```python
from build123d import *

# Parameters (mm, degrees)
F1_DEPTH = 8


with BuildPart() as f1:
    # F0 (on Top) → F1 (new body)
    with BuildSketch(Plane.XY):
        with BuildLine():
            ThreePointArc((0, 14), (-9.899495, -9.899495), (14, 0))
            ThreePointArc((14, 0), (9.899495, 9.899495), (0, 14))
        make_face()
        with BuildLine():
            ThreePointArc((6.347522, 59.107844), (4.032635, 62.692937), (0, 64.089164))
            ThreePointArc((0, 64.089164), (-4.032635, 62.692937), (-6.347522, 59.107844))
            ThreePointArc((-6.347522, 59.107844), (-9.178693, 55.402974), (-13.333366, 53.286307))
            ThreePointArc((-13.333366, 53.286307), (-20.442135, 50.558658), (-24.717154, 44.257954))
            ThreePointArc((-24.717154, 44.257954), (-23.940515, 36.01526), (-18.369188, 29.891087))
            ThreePointArc((-18.369188, 29.891087), (-18.073469, 24.875996), (-22.751722, 26.70699))
            ThreePointArc((-22.751722, 26.70699), (-26.854522, 33.89811), (-34.453795, 37.18387))
            ThreePointArc((-34.453795, 37.18387), (-41.767174, 35.06511), (-46.558052, 29.147159))
            ThreePointArc((-46.558052, 29.147159), (-49.854987, 25.849917), (-54.253408, 24.302181))
            ThreePointArc((-54.253408, 24.302181), (-58.378374, 23.208447), (-60.952417, 19.804641))
            ThreePointArc((-60.952417, 19.804641), (-60.870679, 15.537919), (-58.176392, 12.228476))
            ThreePointArc((-58.176392, 12.228476), (-55.527732, 8.391005), (-54.798526, 3.785589))
            ThreePointArc((-54.798526, 3.785589), (-54.401108, -3.818141), (-49.729836, -9.830951))
            ThreePointArc((-49.729836, -9.830951), (-41.650573, -11.639455), (-34.104504, -8.233282))
            ThreePointArc((-34.104504, -8.233282), (-29.243487, -9.501785), (-32.430525, -13.38526))
            ThreePointArc((-32.430525, -13.38526), (-40.537522, -15.065076), (-46.01077, -21.277058))
            ThreePointArc((-46.01077, -21.277058), (-46.255668, -28.887228), (-42.107825, -35.272372))
            ThreePointArc((-42.107825, -35.272372), (-39.99077, -39.426847), (-39.877972, -44.08827))
            ThreePointArc((-39.877972, -44.08827), (-40.112455, -48.349328), (-37.670666, -51.849223))
            ThreePointArc((-37.670666, -51.849223), (-33.587513, -53.089975), (-29.607466, -51.55023))
            ThreePointArc((-29.607466, -51.55023), (-25.139332, -50.217048), (-20.533985, -50.946684))
            ThreePointArc((-20.533985, -50.946684), (-13.179599, -52.918399), (-6.017575, -50.333815))
            ThreePointArc((-6.017575, -50.333815), (-1.800955, -43.208839), (-2.708555, -34.979535))
            ThreePointArc((-2.708555, -34.979535), (0, -30.748422), (2.708555, -34.979535))
            ThreePointArc((2.708555, -34.979535), (1.800955, -43.208839), (6.017575, -50.333815))
            ThreePointArc((6.017575, -50.333815), (13.179599, -52.918399), (20.533985, -50.946684))
            ThreePointArc((20.533985, -50.946684), (25.139332, -50.217048), (29.607466, -51.55023))
            ThreePointArc((29.607466, -51.55023), (33.587513, -53.089975), (37.670666, -51.849223))
            ThreePointArc((37.670666, -51.849223), (40.112455, -48.349328), (39.877972, -44.08827))
            ThreePointArc((39.877972, -44.08827), (39.99077, -39.426847), (42.107825, -35.272372))
            ThreePointArc((42.107825, -35.272372), (46.255668, -28.887228), (46.01077, -21.277058))
            ThreePointArc((46.01077, -21.277058), (40.537522, -15.065076), (32.430525, -13.38526))
            ThreePointArc((32.430525, -13.38526), (29.243487, -9.501785), (34.104504, -8.233282))
            ThreePointArc((34.104504, -8.233282), (41.650573, -11.639455), (49.729836, -9.830951))
            ThreePointArc((49.729836, -9.830951), (54.401108, -3.818141), (54.798526, 3.785589))
            ThreePointArc((54.798526, 3.785589), (55.527732, 8.391005), (58.176392, 12.228476))
            ThreePointArc((58.176392, 12.228476), (60.870679, 15.537919), (60.952417, 19.804641))
            ThreePointArc((60.952417, 19.804641), (58.378374, 23.208447), (54.253408, 24.302181))
            ThreePointArc((54.253408, 24.302181), (49.854987, 25.849917), (46.558052, 29.147159))
            ThreePointArc((46.558052, 29.147159), (41.767174, 35.06511), (34.453795, 37.18387))
            ThreePointArc((34.453795, 37.18387), (26.854522, 33.89811), (22.751722, 26.70699))
            ThreePointArc((22.751722, 26.70699), (18.073469, 24.875996), (18.369188, 29.891087))
            ThreePointArc((18.369188, 29.891087), (23.940515, 36.01526), (24.717154, 44.257954))
            ThreePointArc((24.717154, 44.257954), (20.442135, 50.558658), (13.333366, 53.286307))
            ThreePointArc((13.333366, 53.286307), (9.178693, 55.402974), (6.347522, 59.107844))
        make_face()
        Polygon((-11.907824, -27.194431), (-13.235514, -39.826555), (-24.8391, -44.992804), (-35.114996, -37.526929), (-33.787306, -24.894804), (-22.18372, -19.728555), align=None, mode=Mode.SUBTRACT)
        with BuildLine():
            ThreePointArc((0, 14), (9.899495, 9.899495), (14, 0))
            ThreePointArc((14, 0), (-9.899495, -9.899495), (0, 14))
        make_face(mode=Mode.SUBTRACT)
        Polygon((22.18372, -19.728555), (33.787306, -24.894804), (35.114996, -37.526929), (24.8391, -44.992804), (13.235514, -39.826555), (11.907824, -27.194431), align=None, mode=Mode.SUBTRACT)
        Polygon((-29.54316, 2.921473), (-41.967304, 0.28064), (-50.466404, 9.719847), (-46.541361, 21.799887), (-34.117218, 24.44072), (-25.618117, 15.001513), align=None, mode=Mode.SUBTRACT)
        Polygon((6.350853, 29), (0, 29), (-6.350853, 29), (-12.701706, 40), (-6.350853, 51), (0, 51), (6.350853, 51), (12.701706, 40), align=None, mode=Mode.SUBTRACT)
        Polygon((25.618117, 15.001513), (34.117218, 24.44072), (46.541361, 21.799887), (50.466404, 9.719847), (41.967304, 0.28064), (29.54316, 2.921473), align=None, mode=Mode.SUBTRACT)
    extrude(amount=F1_DEPTH)


solid = f1.part
```
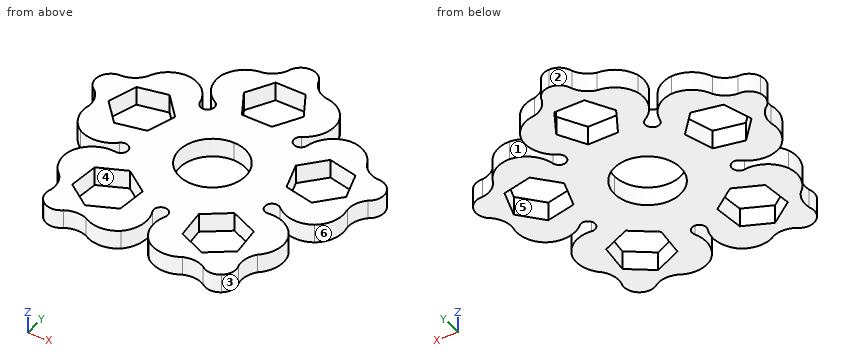
The listing builds one solid part. Answer for the finished solid, in the listing's coordinates (mm). Face numbers are marked on the shaded views. A direction names the side the tool comes from. Round coordinates to 2 decimals unless told otherwise and drop trailing zeros. Write each loop counter-clockwise with the first axis right and the second up, starting at its lowest first coordinate (ties: lowest second). Pieces come first, ordered by that corner, then holes. Notation, with made-up numbers: (64, 66.25) -> (123, 66.25) arc R7 cw to (123, 73.25) -> close; hole circle Ø2 at (85.5, 65). An arc over 180 degrees is marked (long way). Use CSV: the item, a comma, the result in double quotes. Start each with the question number.
(1) Each of these flat-tipped pins is pushed along its axis until it touches: pin 1 (2.5 mm diameter, centred on x = 1.5, z = 4, fed in from +Y); pin 2 (1 mm diameter, centred on x = 41, z = 3.5, fed in from +Y); pin 3 (1.5 mm diameter, centred on y = 8, z = 2, fed in from +X). Where does it stop, or does it pass through?
(2) Section D-D on x = 52 is taken. Give the vertices of the cut face in (y, z), then the cut area to 3 significant figures.
(3) Section A-A on y = 41.5 is taken. Give the vertices of the cut face in (x, z), then the cut area to 3 significant figures.
(4) The mould has two halves that part along X. Classify the marked faces 1, 2, 3 and 4: released by +X, released by -X, zero draft, split by the parting line, or undercut.
(5) Section B-B on y = -4 is taken. Give the vertices of the cut face in (x, z), then the cut area to 3 significant figures.
(6) Section C-C on z = 4.25 is taken. Count the separate pieces of the cut face and the enclosed holes in it, then the cut area to 3 significant figures.
(7) Consider L1, parallel to X at y = 18, z = 5; L2, parallel to X at y = 33.5, z = 1.25; L3, parallel to X at y = -36.5, z = 4. Determine where each line is inside the solid, lowest interval first. Write a range as from..to.
(8) Which of the six approach directions +Z, -Z, +X, -X, +Y, -Y give full straight-line access (tool end or side, diameter ignored) to the marked faces 5 and 6?
A:
1,pin 1,"stops at y = 64.08"
1,pin 2,"stops at y = 35.8"
1,pin 3,"stops at x = 55.68"
2,outline,"(-7.82, 0) -> (24.82, 0) -> (24.82, 8) -> (-7.82, 8) -> close"
2,area,"261 mm²"
3,outline,"(-25.05, 0) -> (-11.84, 0) -> (-11.84, 8) -> (-25.05, 8) -> close; (11.84, 0) -> (25.05, 0) -> (25.05, 8) -> (11.84, 8) -> close"
3,area,"212 mm²"
4,face 1,"undercut"
4,face 2,"released by -X"
4,face 3,"released by +X"
4,face 4,"undercut"
5,outline,"(-54.33, 0) -> (-13.42, 0) -> (-13.42, 8) -> (-54.33, 8) -> close; (13.42, 0) -> (54.33, 0) -> (54.33, 8) -> (13.42, 8) -> close"
5,area,"655 mm²"
6,separate pieces,"1"
6,enclosed holes,"6"
6,area,"6,460 mm²"
7,L1,"x = -61.27..-47.78, -28.32..28.32, 47.78..61.27"
7,L2,"x = -43.69..-26.43, -22.47..-8.95, 8.95..22.47, 26.43..43.69"
7,L3,"x = -41.23..-35.01, -12.89..-2.12, 2.12..12.89, 35.01..41.23"
8,face 5,"+Z, -Z"
8,face 6,"+Z, -Z, +X"
